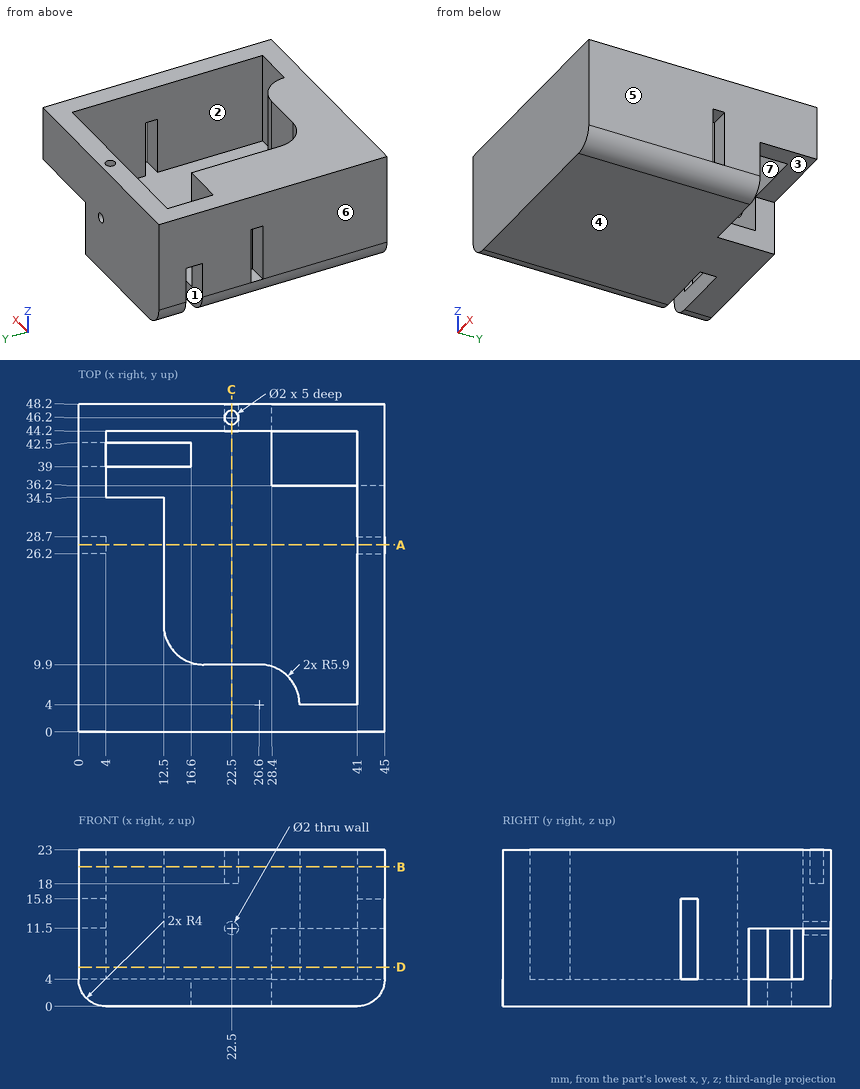
Part print with two shaded views. Sizes in mm from the minimum x, y, z corner. A direction names the side the tool comes from. Round coordinates to 2 decimals unless told otherwise and drop trailing zeros. Order: outer loops, then holes, each group sorted by start corner. A loop starts at its lowest first (then second) coordinate and runs counter-clockwise, first axis right, second up. Notation, with made-up numbers: M 14,2 L 37,2 A22 ccw 37,25 Z; hole C -0.5,42 d4. An arc over 180 degrees is marked long. Answer in a Markdown table with one row per item. Add a question column.
Q1. Wall check: L1, parallel to Y at x = 22.5, z = 21.3; L2, parallel to X at y = 42, z = 21.5; L3, parallel to Z at x = 22.5, y = 47.25. Give the ranges that are in metal, low to high. Write a range as from..to.
Q2. Cut at D-D on z = 5.75. Give the cut face in (x, y), and give its area (3 significant figures).
Q3. Mould opens along X. For the marked faces 5, 6 and 7 say: +X half, -X half, draft (parallel to the pull), parting line (faces both ways), or undercut.
Q4. Cut at A-A on y = 27.5. Give the cut face in (x, z), and give its area (3 significant figures).
Q5. 3-axis set-ups, long thin cutter, end or side, ignore diameter. For the marked faces 1, 2, 3 and 4: which of +Z, -Z, +X, -X, +Y, -Y reach the whole face in a straight line?
Q6. Cut at C-C on x = 22.5. Give the cut face in (y, z), and give its area (3 significant figures).
Q7. Pin check, flat tips, straight feed: pin 1 (4.5 mm diameter, centred on x = 42, z = 12.5, fed in from -Y); pin 2 (1.2 mm diameter, centred on x = 43.5, y = 27, fed in from -Z); pin 3 (6 mm diameter, centred on x = 36.5, y = 45, fed in from -Z); pin 4 (1 mm diameter, centred on x = 22.5, y = 46, fed in from +Z). Stop position of each tip, or through.
Q8. Cut at B-B on z = 20.5. Give the cut face in (x, y).
Established:
| question | item | result |
|---|---|---|
| 1 | L1 | y = 0..9.9, 44.2..45.2, 47.2..48.2 |
| 1 | L2 | x = 0..4, 41..45 |
| 1 | L3 | z = 0..10.5, 12.5..23 |
| 2 | outline | M 0,0 L 45,0 L 45,26.2 L 41,26.2 L 41,4 L 32.5,4 A5.9 ccw 26.6,9.9 L 18.4,9.9 A5.9 cw 12.5,15.8 L 12.5,34.5 L 4,34.5 L 4,39 L 0,39 L 0,28.7 L 4,28.7 L 4,26.2 L 0,26.2 Z; M 0,42.5 L 4,42.5 L 4,44.2 L 28.4,44.2 L 28.4,48.2 L 0,48.2 Z; M 41,28.7 L 45,28.7 L 45,36.2 L 41,36.2 Z |
| 2 | area | 926 mm2 |
| 3 | face 5 | +X half |
| 3 | face 6 | -X half |
| 3 | face 7 | undercut |
| 4 | outline | M 0,4 A4 ccw 4,0 L 41,0 A4 ccw 45,4 L 12.5,4 L 12.5,23 L 0,23 L 0,15.8 L 4,15.8 L 4,4 Z; M 41,15.8 L 45,15.8 L 45,23 L 41,23 Z |
| 4 | area | 392 mm2 |
| 5 | face 1 | -Z, -X |
| 5 | face 2 | +Z |
| 5 | face 3 | -Z, +X, +Y |
| 5 | face 4 | -Z, +X, -X, +Y, -Y |
| 6 | outline | M 0,0 L 48.2,0 L 48.2,10.5 L 44.2,10.5 L 44.2,4 L 9.9,4 L 9.9,23 L 0,23 Z; M 44.2,12.5 L 48.2,12.5 L 48.2,23 L 47.2,23 L 47.2,18 L 45.2,18 L 45.2,23 L 44.2,23 Z |
| 6 | area | 439 mm2 |
| 7 | pin 1 | stops at y = 0 |
| 7 | pin 2 | stops at z = 0.48 |
| 7 | pin 3 | stops at z = 11.5 |
| 7 | pin 4 | stops at z = 18 |
| 8 | outline | M 0,0 L 45,0 L 45,48.2 L 0,48.2 Z; hole M 4,34.5 L 12.5,34.5 L 12.5,15.8 A5.9 ccw 18.4,9.9 L 26.6,9.9 A5.9 cw 32.5,4 L 41,4 L 41,44.2 L 4,44.2 Z; hole C 22.5,46.2 d2 |
